Geometry: final body of the model. Coordinates: model frame, mm. Give positions to 0.01 mm unless a question says otherwise; leave off trailing zeros. Write each loop counter-clockwise with the first axis right and the second up, starting at its lowest first coordinate (ties: lowest second). Pieces come first, ordered by that corner, then holes.
Q1. Pin query (flat end, axial travel): pin 1 Ø1.5 at (y, z) = (1.5, 87.5) entering from +X; pin 2 Ø1 at (y, z) = (2.5, 10.5) entering from -X; pin 3 Ø2 at (x, y) = (42, 1) entering from -Z. Return the tip coordinate at first contact, or that it passes through.
Q2. Section D-D (z = 44.5). Return the cut outline in (x, y).
Q3. Section C-C (y = 1.85). State how many separate pieces and enclosed holes the cut face has, plus the area to 3 significant figures.
Q4. Line query: line 1 (X direction, y = 1.05, z = 10.5); line 2 (X direction, y = 2.75, z = 105.2); line 3 (X direction, y = 1.25, z = -10.5). Output: solid intervals per line, ascending.
Q5. Section B-B (z = -10.5). Return the cut outline in (x, y).
Q6. Section A-A (x = 41). Return the cut outline in (y, z).
from build123d import *

# Parameters (mm, degrees)
SKETCH2_R           = 1.7
SKETCH2_R_2         = 1.1
BOSS_EXTRUDE1_DEPTH = 4
FILLET1_R           = 5


with BuildPart() as part:
    # Sketch2 → Boss-Extrude1 (new body)
    with BuildSketch(Plane(origin=(0, 0, 0), x_dir=(1, 0, 0), z_dir=(0, 1, 0))):
        with BuildLine():
            Line((-33, -13), (33, -13))
            ThreePointArc((33, -13), (34.060660172, -12.560660172), (34.5, -11.5))
            Line((34.5, -11.5), (34.5, -10.5))
            ThreePointArc((34.5, -10.5), (34.939339828, -9.439339828), (36, -9))
            Line((36, -9), (55.5, -9))
            ThreePointArc((55.5, -9), (56.914213562, -8.414213562), (57.5, -7))
            Line((57.5, -7), (57.5, 3))
            ThreePointArc((57.5, 3), (56.914213562, 4.414213562), (55.5, 5))
            Line((55.5, 5), (51.5, 5))
            ThreePointArc((51.5, 5), (50.085786438, 5.585786438), (49.5, 7))
            Line((49.5, 7), (49.5, 14))
            ThreePointArc((49.5, 14), (50.085786438, 15.414213562), (51.5, 16))
            Line((51.5, 16), (62.5, 16))
            ThreePointArc((62.5, 16), (63.914213562, 15.414213562), (64.5, 14))
            Line((64.5, 14), (64.5, -13))
            Line((64.5, -13), (64.5, -14.5))
            ThreePointArc((64.5, -14.5), (64.060660172, -15.560660172), (63, -16))
            Line((63, -16), (36, -16))
            ThreePointArc((36, -16), (34.939339828, -16.439339828), (34.5, -17.5))
            Line((34.5, -17.5), (34.5, -21.5))
            ThreePointArc((34.5, -21.5), (34.060660172, -22.560660172), (33, -23))
            Line((33, -23), (17.5, -23))
            ThreePointArc((17.5, -23), (13.964466094, -24.464466094), (12.5, -28))
            Line((12.5, -28), (12.5, -56.5))
            Line((12.5, -56.5), (12.5, -71.5))
            ThreePointArc((12.5, -71.5), (15.428932188, -78.571067812), (22.5, -81.5))
            Line((22.5, -81.5), (55, -81.5))
            ThreePointArc((55, -81.5), (62.071067812, -84.428932188), (65, -91.5))
            Line((65, -91.5), (65, -146.5))
            Line((65, -146.5), (-65, -146.5))
            Line((-65, -146.5), (-65, -91.5))
            ThreePointArc((-65, -91.5), (-62.071067812, -84.428932188), (-55, -81.5))
            Line((-55, -81.5), (-25, -81.5))
            Line((-25, -81.5), (-22.5, -81.5))
            ThreePointArc((-22.5, -81.5), (-15.428932188, -78.571067812), (-12.5, -71.5))
            Line((-12.5, -71.5), (-12.5, -56.5))
            Line((-12.5, -56.5), (-12.5, -28))
            ThreePointArc((-12.5, -28), (-13.964466094, -24.464466094), (-17.5, -23))
            Line((-17.5, -23), (-33, -23))
            ThreePointArc((-33, -23), (-34.060660172, -22.560660172), (-34.5, -21.5))
            Line((-34.5, -21.5), (-34.5, -17.5))
            ThreePointArc((-34.5, -17.5), (-34.939339828, -16.439339828), (-36, -16))
            Line((-36, -16), (-63, -16))
            ThreePointArc((-63, -16), (-64.060660172, -15.560660172), (-64.5, -14.5))
            Line((-64.5, -14.5), (-64.5, -13))
            Line((-64.5, -13), (-64.5, 14))
            ThreePointArc((-64.5, 14), (-63.914213562, 15.414213562), (-62.5, 16))
            Line((-62.5, 16), (-51.5, 16))
            ThreePointArc((-51.5, 16), (-50.085786438, 15.414213562), (-49.5, 14))
            Line((-49.5, 14), (-49.5, 7))
            ThreePointArc((-49.5, 7), (-50.085786438, 5.585786438), (-51.5, 5))
            Line((-51.5, 5), (-55.5, 5))
            ThreePointArc((-55.5, 5), (-56.914213562, 4.414213562), (-57.5, 3))
            Line((-57.5, 3), (-57.5, -7))
            ThreePointArc((-57.5, -7), (-56.914213562, -8.414213562), (-55.5, -9))
            Line((-55.5, -9), (-36, -9))
            ThreePointArc((-36, -9), (-34.939339828, -9.439339828), (-34.5, -10.5))
            Line((-34.5, -10.5), (-34.5, -11.5))
            ThreePointArc((-34.5, -11.5), (-34.060660172, -12.560660172), (-33, -13))
        make_face()
        with Locations(Location((59, 10.5, 0), (0, 0, 270))):
            Circle(SKETCH2_R, mode=Mode.SUBTRACT)
        with Locations(Location((-59, 10.5, 0), (0, 0, 90))):
            Circle(SKETCH2_R, mode=Mode.SUBTRACT)
        with Locations(Location((-59, -10.5, 0), (0, 0, 270))):
            Circle(SKETCH2_R, mode=Mode.SUBTRACT)
        with Locations(Location((59, -10.5, 0), (0, 0, 90))):
            Circle(SKETCH2_R, mode=Mode.SUBTRACT)
        with Locations(Location((-60.8, -105.2, 0), (0, 0, 270))):
            Circle(SKETCH2_R_2, mode=Mode.SUBTRACT)
        with Locations(Location((-60.8, -122.8, 0), (0, 0, 90))):
            Circle(SKETCH2_R_2, mode=Mode.SUBTRACT)
        with Locations(Location((60.8, -122.8, 0), (0, 0, 270))):
            Circle(SKETCH2_R_2, mode=Mode.SUBTRACT)
        with Locations(Location((60.8, -105.2, 0), (0, 0, 90))):
            Circle(SKETCH2_R_2, mode=Mode.SUBTRACT)
    extrude(amount=BOSS_EXTRUDE1_DEPTH)

    # Fillet1
    fillet1_edges = [part.edges().sort_by_distance(p)[0] for p in [
        (65, 2, 146.5),
        (-65, 2, 146.5),
    ]]
    fillet(fillet1_edges, radius=FILLET1_R)


solid = part.part
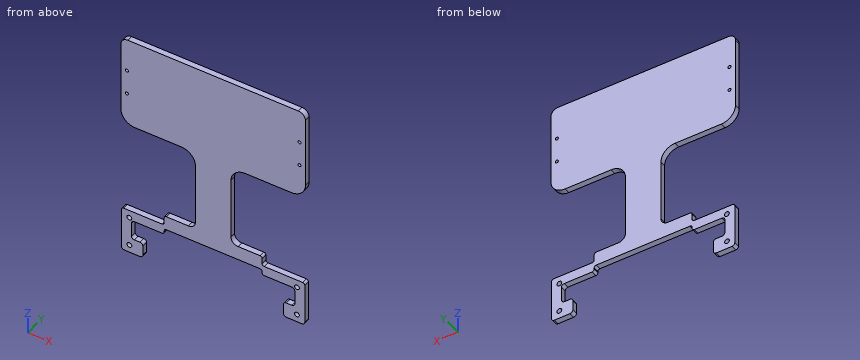
Computed:
1. pin 1: stops at x = 64.46
1. pin 2: stops at x = -64.5
1. pin 3: stops at z = 9
2. outline: (-12.5, 0) - (12.5, 0) - (12.5, 4) - (-12.5, 4) - close
3. separate pieces: 1
3. enclosed holes: 8
3. area: 11,500 mm2
4. line 1: x = -64.5 to -60.7, -57.3 to -34.5, 34.5 to 57.3, 60.7 to 64.5
4. line 2: x = -65 to -61.9, -59.7 to 59.7, 61.9 to 65
4. line 3: x = -64.5 to -60.7, -57.3 to -49.5, 49.5 to 57.3, 60.7 to 64.5
5. outline: (-64.5, 0) - (-60.7, 0) - (-60.7, 4) - (-64.5, 4) - close; (-57.3, 0) - (-49.5, 0) - (-49.5, 4) - (-57.3, 4) - close; (49.5, 0) - (57.3, 0) - (57.3, 4) - (49.5, 4) - close; (60.7, 0) - (64.5, 0) - (64.5, 4) - (60.7, 4) - close
6. outline: (0, 9) - (4, 9) - (4, 16) - (0, 16) - close; (0, 81.5) - (4, 81.5) - (4, 146.5) - (0, 146.5) - close
